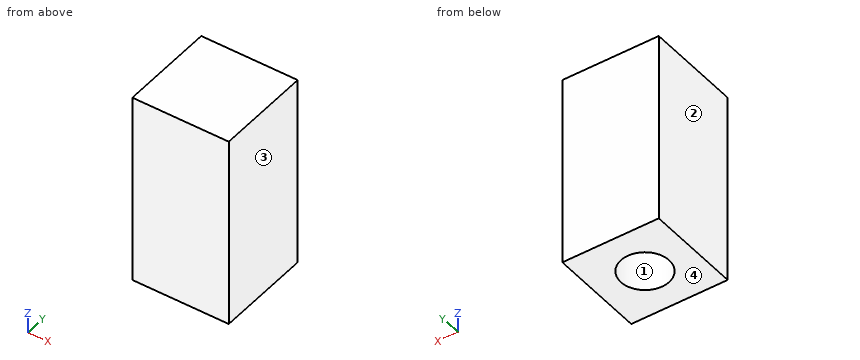
```python
from build123d import *

# Parameters (mm, degrees)
SKETCH1_W           = 20
SKETCH1_H           = 20
BOSS_EXTRUDE1_DEPTH = 40
SKETCH2_R           = 5
CUT_EXTRUDE1_DEPTH  = 10


with BuildPart() as part:
    # Sketch1 → Boss-Extrude1 (new body)
    with BuildSketch(Plane.XY):
        with Locations((0.569105691, -2.256097561)):
            Rectangle(SKETCH1_W, SKETCH1_H)
    extrude(amount=BOSS_EXTRUDE1_DEPTH)

    # Sketch2 → Cut-Extrude1 (cut, symmetric)
    with BuildSketch(Plane(origin=(0, 0, 0), x_dir=(-1, 0, 0), z_dir=(0, 0, -1))):
        with Locations((-0.569105691, -2.256097561)):
            Circle(SKETCH2_R)
    extrude(amount=CUT_EXTRUDE1_DEPTH, both=True, mode=Mode.SUBTRACT)


solid = part.part
```
Verification items for the finished model (mm, model axes). Face numbers are marked on the shaded views. Give positions to 0.01 mm unless a question says otherwise; leave off trailing zeros. Write each loop counter-clockwise with the first axis right and the second up, starting at its lowest first coordinate (ties: lowest second). Pieces come first, ordered by that corner, then holes. Notation, with made-up numbers: (66, -21.5) - (79, -21.5) arc R21 ccw to (79, -9.5) - close; hole circle Ø8 at (34.25, 53). An arc over 180 degrees is marked (long way). Put each result on its own line as item: value.
Q1. Scan lines: probe 1 along Z at (x, y) = (1, -4.75); probe 2 along X at (y, z) = (-4, 8); probe 3 along Y at (x, z) = (-0.75, 8). Record each from-to range of solid material in increasing order. Write a range as from..to.
Result:
probe 1: 10..40
probe 2: -9.43..-4.12, 5.26..10.57
probe 3: -12.26..-7.08, 2.57..7.74
Q2. Mould release check, pull along X, two halves, no side actions. Record for the marked faces 1, 2, 3 and 4: released by +X, released by -X, zero draft, split by the parting line, or undercut.
Result:
face 1: undercut
face 2: released by -X
face 3: released by +X
face 4: zero draft
Q3. Section check A-A on x = 4.5. Record the cut outline in (y, z), and give its area (3 significant figures).
Result:
outline: (-12.26, 0) - (-5.35, 0) - (-5.35, 10) - (0.83, 10) - (0.83, 0) - (7.74, 0) - (7.74, 40) - (-12.26, 40) - close
area: 738 mm2
Q4. Section check C-C on z = 5.5. Record the cut outline in (x, y), and give its area (3 significant figures).
Result:
outline: (-9.43, -12.26) - (10.57, -12.26) - (10.57, 7.74) - (-9.43, 7.74) - close; hole circle Ø10 at (0.57, -2.26)
area: 321 mm2
Q5. Section check B-B on y = 1.5. Record the cut outline in (x, z).
Result:
outline: (-9.43, 0) - (-2.73, 0) - (-2.73, 10) - (3.87, 10) - (3.87, 0) - (10.57, 0) - (10.57, 40) - (-9.43, 40) - close
